Build history of the part. All positions in model axes, mm. Face numbers are marked on the shaded views. A direction names the side the tool comes from. Round coordinates to 2 decimals unless told otherwise and drop trailing zeros. Order: outer loops, then holes, each group sorted by start corner. A loop starts at its lowest first (then second) coordinate and runs counter-clockwise, first axis right, second up. Notation, with made-up numbers: (79.5, 86.5) -> (90.5, 86.5) arc R10 ccw to (90.5, 102.5) -> close; hole circle Ø2 at (43, -33.5). An arc over 180 degrees is marked (long way). Use a Markdown table: item, result. Add a question column.
Item 1: Slice it at A-A, the plane z = -3.5. Give the cut face in (x, y).
Item 2: Slice it at B-B, the plane y = -9. Give the cut face in (x, z) (3 decimals).
Item 3: 3-axis set-ups, long thin cutter, end or side, ignore diameter. For the marked faces 1 and 2: which of +Z, -Z, +X, -X, +Y, -Y reach the whole face in a straight line?
Item 4: Probe L1, parallel to Z at x = -1.2, y = -7 (3 decimals); L2, parallel to Y at x = -1.05, z = -3.75; L3, parallel to Y at x = 0.8, z = 2.5. List the from-to ranges inside material, lowest first.
Item 5: Slice it at D-D, the plane z = -1.75. Give the cut face in (x, y), plus the area to 3 significant figures.
Item 6: Pin check, flat tips, straight feed: pin 1 (3 mm diameter, centred on y = 1, z = -4, fed in from -X); pin 2 (2 mm diameter, centred on x = -0.5, z = -2, fed in from +Y); pin 3 (5 mm diameter, centred on y = -5, z = 2, fed in from +X); pin 4 (4 mm diameter, centred on y = -8.5, z = -3, fed in from -X). Stop position of each tip, or through.
Item 7: Slice it at C-C, the plane x = 0. Give the cut face in (y, z).
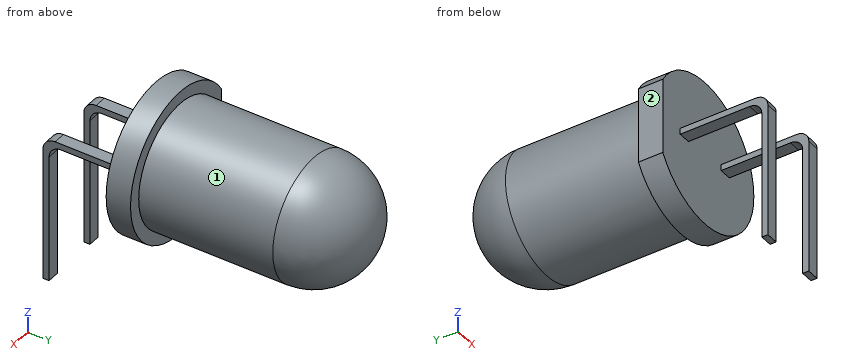
from build123d import *

# Parameters (mm, degrees)
SKETCH2_W           = 0.5
SKETCH2_H           = 0.25
EXTRUDE1_DEPTH      = 30
SKETCH3_W           = 0.5
SKETCH3_H           = 10
EXTRUDE3_DEPTH      = 2
EXTRUDE3_DEPTH_BACK = 2
SKETCH4_W           = 0.5
SKETCH4_H           = 3.5
EXTRUDE4_DEPTH      = 2
BOSS_EXTRUDE1_DEPTH = 3
CUT_EXTRUDE1_DEPTH  = 10
FILLET1_R           = 0.5


with BuildPart() as part:
    # Sketch1 → Revolve1 (revolve)
    with BuildSketch(Plane.XY):
        with BuildLine():
            Line((0, 2.5), (0, -5.5))
            Line((0, -5.5), (0, -6.5))
            Line((0, -6.5), (3, -6.5))
            Line((3, -6.5), (3, -5.5))
            Line((3, -5.5), (2.5, -5.5))
            Line((2.5, -5.5), (2.5, 0))
            ThreePointArc((2.5, 0), (1.767766953, 1.767766953), (0, 2.5))
        make_face()
    revolve(axis=Axis((0, 40.48125, 0), (0, -1, 0)))

    # Sketch2 → Extrude1 (add)
    with BuildSketch(Plane.XZ.offset(6.5)):
        with Locations((1.25, 0)):
            Rectangle(SKETCH2_W, SKETCH2_H)
        with Locations((-1.25, 0)):
            Rectangle(SKETCH2_W, SKETCH2_H)
    extrude(amount=EXTRUDE1_DEPTH)

    # Sketch3 → Extrude3 (cut, two sides)
    with BuildSketch(Plane.XY) as extrude3_sk:
        with Locations((-1.25, -31.5)):
            Rectangle(SKETCH3_W, SKETCH3_H)
    extrude(amount=EXTRUDE3_DEPTH, mode=Mode.SUBTRACT)
    extrude(extrude3_sk.sketch, amount=-EXTRUDE3_DEPTH_BACK, mode=Mode.SUBTRACT)

    # Sketch4 → Extrude4 (cut)
    with BuildSketch(Plane.XZ.offset(6.5)):
        with Locations((-2.817517664, 0)):
            Rectangle(SKETCH4_W, SKETCH4_H)
    extrude(amount=-EXTRUDE4_DEPTH, mode=Mode.SUBTRACT)

    # Sketch5 → Boss-Extrude1 (add)
    with BuildSketch(Plane.ZY.offset(1.5)):
        Polygon((0.125, -10.097548576), (-5.875, -10.097548576), (-5.875, -9.847548576), (-0.125, -9.847548576), align=None)
    extrude(amount=-BOSS_EXTRUDE1_DEPTH)

    # Sketch6 → Cut-Extrude1 (cut)
    with BuildSketch(Plane.XY.offset(0.125)):
        Polygon((-1, -8.951862253), (1, -8.951862253), (1, -10.097548576), (1.5, -10.097548576), (1.5, -37.452172459), (-1.5, -37.452172459), (-1.5, -10.097548576), (-1, -10.097548576), align=None)
    extrude(amount=-CUT_EXTRUDE1_DEPTH, mode=Mode.SUBTRACT)

    # Fillet1
    fillet1_edges = [part.edges().sort_by_distance(p)[0] for p in [
        (1.25, -10.097548576, 0.125),
        (-1.25, -10.097548576, 0.125),
        (-1.25, -9.847548576, -0.125),
        (1.25, -9.847548576, -0.125),
    ]]
    fillet(fillet1_edges, radius=FILLET1_R)


solid = part.part
Check sheet entries:
| question | item | result |
|---|---|---|
| 1 | outline | (-1.5, -10.1) -> (-1, -10.1) -> (-1, -9.85) -> (-1.5, -9.85) -> close; (1, -10.1) -> (1.5, -10.1) -> (1.5, -9.85) -> (1, -9.85) -> close |
| 2 | outline | (-1.5, -0.125) -> (-1, -0.125) -> (-1, 0.125) -> (-1.5, 0.125) -> close; (1, -0.125) -> (1.5, -0.125) -> (1.5, 0.125) -> (1, 0.125) -> close |
| 3 | face 1 | +Y |
| 3 | face 2 | +Z, -Z, -X, +Y, -Y |
| 4 | L1 | -0.125 to 0.125 |
| 4 | L2 | -10.1 to -9.85 |
| 4 | L3 | -6.5 to -5.5 |
| 5 | outline | (-2.44, -6.5) -> (2.44, -6.5) -> (2.44, -5.5) -> (1.79, -5.5) -> (1.79, 0) arc R1.79 ccw to (-1.79, 0) -> (-1.79, -5.5) -> (-2.44, -5.5) -> close; (-1.5, -10.1) -> (-1, -10.1) -> (-1, -9.85) -> (-1.5, -9.85) -> close; (1, -10.1) -> (1.5, -10.1) -> (1.5, -9.85) -> (1, -9.85) -> close |
| 5 | area | 29.8 mm2 |
| 6 | pin 1 | through |
| 6 | pin 2 | y = 2.26 |
| 6 | pin 3 | x = 3 |
| 6 | pin 4 | x = -1.5 |
| 7 | outline | (-6.5, -3) -> (-5.5, -3) -> (-5.5, -2.5) -> (0, -2.5) arc R2.5 ccw to (0, 2.5) -> (-5.5, 2.5) -> (-5.5, 3) -> (-6.5, 3) -> close |
